from build123d import *

# Parameters (mm, degrees)
SKETCH1_R                  = 45
SKETCH1_R_2                = 5
BOSS_EXTRUDE1_DEPTH        = 8
F_4_3_4_3_DIAMETER_HOLE1_D = 4.3
SKETCH6_R                  = 30.1
SKETCH6_R_2                = 19.9
CUT_EXTRUDE2_DEPTH         = 1.5
SKETCH8_R                  = 24
SKETCH8_R_2                = 12.5
CUT_EXTRUDE3_DEPTH         = 3
SKETCH9_R                  = 24
SKETCH9_R_2                = 14.5
CUT_EXTRUDE4_DEPTH         = 0.6


with BuildPart() as part:
    # Sketch1 → Boss-Extrude1 (new body)
    with BuildSketch(Plane(origin=(0, 0, 0), x_dir=(1, 0, 0), z_dir=(0, 1, 0))):
        with Locations(Location((0, 0, 0), (0, 0, 270))):
            Circle(SKETCH1_R)
        with Locations(Location((0, 36.5, 0), (0, 0, 270))):
            Circle(SKETCH1_R_2, mode=Mode.SUBTRACT)
        with Locations(Location((34.713562845, 11.279120295, 0), (0, 0, 270))):
            Circle(SKETCH1_R_2, mode=Mode.SUBTRACT)
        with Locations(Location((21.454161709, -29.529120295, 0), (0, 0, 270))):
            Circle(SKETCH1_R_2, mode=Mode.SUBTRACT)
        with Locations(Location((-21.454161709, -29.529120295, 0), (0, 0, 270))):
            Circle(SKETCH1_R_2, mode=Mode.SUBTRACT)
        with Locations(Location((-34.713562845, 11.279120295, 0), (0, 0, 270))):
            Circle(SKETCH1_R_2, mode=Mode.SUBTRACT)
    extrude(amount=BOSS_EXTRUDE1_DEPTH)

    # Ø4.3 (4.3) Diameter Hole1 (through all)
    with Locations(Plane(origin=(0, 8, 0), x_dir=(1, 0, 0), z_dir=(0, 1, 0))):
        with Locations((-7.60845213, -2.472135955), (-4.702282018, 6.472135955), (4.702282018, 6.472135955), (7.60845213, -2.472135955), (0, -8)):
            Hole(F_4_3_4_3_DIAMETER_HOLE1_D / 2)

    # Sketch6 → Cut-Extrude2 (cut)
    with BuildSketch(Plane.XZ):
        with Locations(Location((0, 0, 0), (0, 0, 270))):
            Circle(SKETCH6_R)
        with Locations(Location((0, 0, 0), (0, 0, 270))):
            Circle(SKETCH6_R_2, mode=Mode.SUBTRACT)
    extrude(amount=-CUT_EXTRUDE2_DEPTH, mode=Mode.SUBTRACT)

    # Sketch8 → Cut-Extrude3 (cut)
    with BuildSketch(Plane(origin=(0, 8, 0), x_dir=(1, 0, 0), z_dir=(0, 1, 0))):
        with Locations(Location((0, 0, 0), (0, 0, 270))):
            Circle(SKETCH8_R)
        with Locations(Location((0, 0, 0), (0, 0, 270))):
            Circle(SKETCH8_R_2, mode=Mode.SUBTRACT)
    extrude(amount=-CUT_EXTRUDE3_DEPTH, mode=Mode.SUBTRACT)

    # Sketch9 → Cut-Extrude4 (cut)
    with BuildSketch(Plane(origin=(0, 5, 0), x_dir=(1, 0, 0), z_dir=(0, 1, 0))):
        with Locations(Location((0, 0, 0), (0, 0, 270))):
            Circle(SKETCH9_R)
        with Locations(Location((0, 0, 0), (0, 0, 270))):
            Circle(SKETCH9_R_2, mode=Mode.SUBTRACT)
    extrude(amount=-CUT_EXTRUDE4_DEPTH, mode=Mode.SUBTRACT)


solid = part.part
The listing builds one solid part. Answer for the finished solid, in the listing's coordinates (mm). A direction names the side the tool comes from. Round coordinates to 2 decimals unless told otherwise and drop trailing zeros. Write each loop counter-clockwise with the first axis right and the second up, starting at its lowest first coordinate (ties: lowest second). Pieces come first, ordered by that corner, then holes. Notation, with made-up numbers: (-25, 15.5) - (3, 15.5) arc R37 cw to (3, 51.5) - close; hole circle Ø4 at (-9, 12.5). An arc over 180 degrees is marked (long way). Use a Markdown table: item, result. Add a question column.
1. Flat-ended cylindrical pins translate along their axes: P1, Ø3, axis at x = 15.5, y = 1.5, coming from the +Z side; P2, Ø13, axis at x = -34.71, z = -11.28, coming from the +Y side; P3, Ø4, axis at x = 32.5, y = 1.5, coming from the +Z side; P4, Ø3, axis at y = 4.5, z = -16, coming from the -X side. Find the tip coordinate at first contact, or state that the pin passes through.
2. A tool of negligible diameter and unlimited length cuts with its end or side. For faces 1 (the face through (-5.554, 4.704, 13.394)), 2 (the face through (0.28, 3.94, 5.87)), 3 (the face through (-20, 1.5, -6)), from which of +Z, -Z, +X, -X, +Y, -Y can it reach the whole face along a straight path? Write none if from no direction.
3. The part is cut by section C-C (z = -36.5). Write down the section's boundary in (x, y).
4. For a pull along X with two mould halves and no side action, classify faces 4 (the face through (9.193, 3.944, 1.019)), 5 (the face through (-17.235, 3.944, 41.569)), 6 (the face through (-29.384, 0.74, 6.525)), 7 (the face through (-9, 0, 29)) as +X half, -X half, draft (parallel to the pull), parting line (faces both ways), or undercut.
5. Consider line 1 (X direction, y = 7.25, z = 26.5); line 2 (Z direction, x = 7.5, y = 4.5); line 3 (Z direction, x = 30.5, y = 3). Determine where each line is inside the solid, lowest interval first.
6. The part is cut by section A-A (x = 0). Give the number of separate pieces and of enclosed holes in the cut face, and give its area (3 significant figures).
7. The part is cut by section B-B (z = 8). Write down the section's boundary in (x, y).
Reported:
| question | item | result |
|---|---|---|
| 1 | P1 | z = 42.77 |
| 1 | P2 | y = 8 |
| 1 | P3 | z = 33.09 |
| 1 | P4 | x = -42.6 |
| 2 | face 1 | +Y |
| 2 | face 2 | +Y, -Y |
| 2 | face 3 | -Y |
| 3 | outline | (-26.32, 0) - (-5, 0) - (-5, 8) - (-26.32, 8) - close; (5, 0) - (26.32, 0) - (26.32, 8) - (5, 8) - close |
| 4 | face 4 | undercut |
| 4 | face 5 | parting line |
| 4 | face 6 | undercut |
| 4 | face 7 | draft |
| 5 | line 1 | -36.37 to -25.43, -17.48 to 17.48, 25.43 to 36.37 |
| 5 | line 2 | -44.37 to -22.8, -12.41 to 0.32, 4.62 to 12.41, 22.8 to 44.37 |
| 5 | line 3 | -33.09 to -13.97, -8.59 to 33.09 |
| 6 | separate pieces | 3 |
| 6 | enclosed holes | 0 |
| 6 | area | 495 mm^2 |
| 7 | outline | (-44.28, 0) - (-29.02, 0) - (-29.02, 1.5) - (-18.22, 1.5) - (-18.22, 0) - (-2.15, 0) - (-2.15, 8) - (-9.6, 8) - (-9.6, 5) - (-12.09, 5) - (-12.09, 4.4) - (-22.63, 4.4) - (-22.63, 8) - (-44.28, 8) - close; (2.15, 0) - (18.22, 0) - (18.22, 1.5) - (29.02, 1.5) - (29.02, 0) - (44.28, 0) - (44.28, 8) - (22.63, 8) - (22.63, 4.4) - (12.09, 4.4) - (12.09, 5) - (9.6, 5) - (9.6, 8) - (2.15, 8) - close |
